Study the drawing (mm; zero at the part's minimum x, y, z) and answer. A direction names the side the tool comes from. Give positions to 0.01 mm unless a question says otherwise; leave off trailing zeros. Write each loop counter-clockwise with the first axis right and the second up, starting at its lowest first coordinate (ties: lowest second). Pieces come first, ordered by that corner, then holes. Notation, with made-up numbers: M 1,10 L 40,10 A14 cw 40,28 Z; hole C -0.75,-25 d11. An arc over 180 degrees is marked long. Use a Markdown table: item, result. Add a question column.
Item 1: Given P1, Ø8, axis at x = 58, z = 9, coming from the -Y side; P2, Ø4, axis at y = 15, z = 13, coming from the -X side, each flat-ended and moving along its own axis, determine where each tip first touches the part or whether it passes through.
Item 2: Consider probe 1 along Z at (x, y) = (50.5, 27); probe 2 along Y at (x, z) = (58.5, 17.75). Determine where each line is inside the solid, lowest interval first. Write a range as [from, to].
Item 3: For the marked faces 1 and 2, determine the directions among +Z, -Z, +X, -X, +Y, -Y from which every point of the face is accessible in a straight line to the end or side of a thin tool.
Item 4: A cutting plane is placed at A-A on y = 44. Determine the outline of the cut face in (x, z).
Item 5: A cutting plane is placed at C-C on x = 31.5. Determine the outline of the cut face in (y, z), then the cut area to 3 significant figures.
Item 6: A cutting plane is placed at B-B on x = 48.5. Determine the outline of the cut face in (y, z) (1 decimal).
Item 7: A cutting plane is placed at D-D on z = 6.5. Determine the outline of the cut face in (x, y), then the cut area to 3 significant figures.
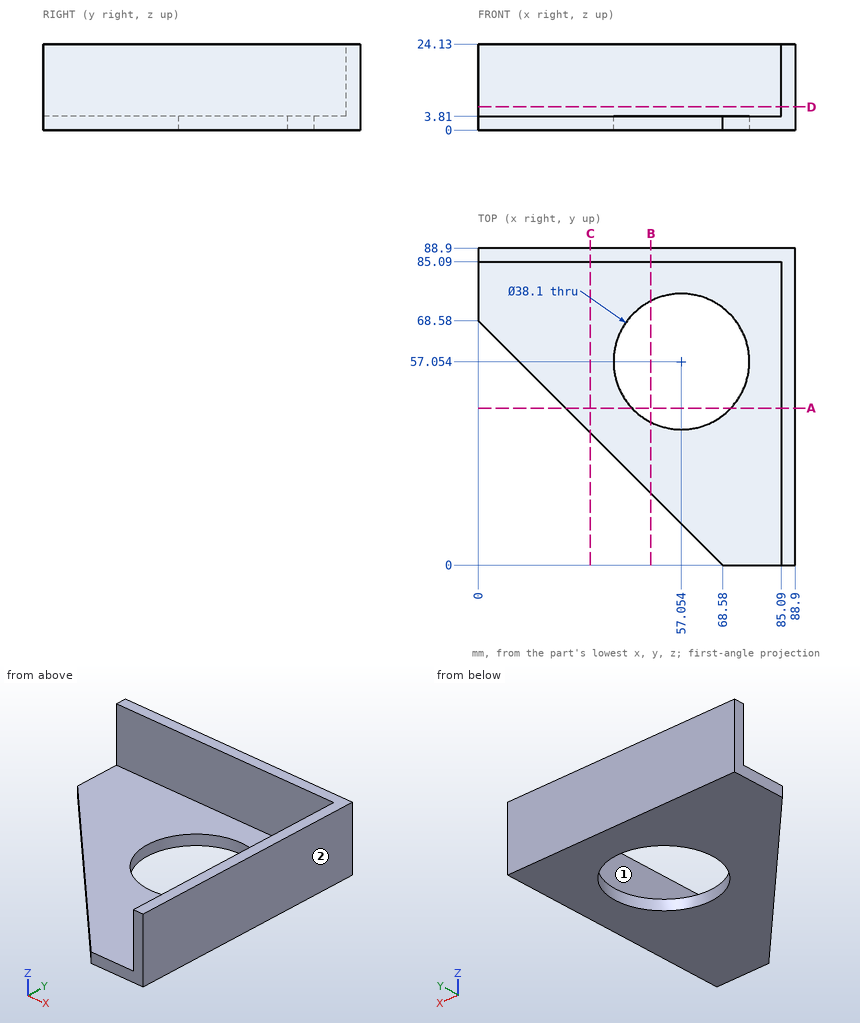
Filled in:
| question | item | result |
|---|---|---|
| 1 | P1 | y = 85.09 |
| 1 | P2 | x = 85.09 |
| 2 | probe 1 | [0, 3.81] |
| 2 | probe 2 | [85.09, 88.9] |
| 3 | face 1 | +Z, -X, -Y |
| 3 | face 2 | +Z, -Z, +X, +Y, -Y |
| 4 | outline | M 24.58,0 L 43.18,0 L 43.18,3.81 L 24.58,3.81 Z; M 70.93,0 L 88.9,0 L 88.9,24.13 L 85.09,24.13 L 85.09,3.81 L 70.93,3.81 Z |
| 5 | outline | M 37.08,0 L 88.9,0 L 88.9,24.13 L 85.09,24.13 L 85.09,3.81 L 37.08,3.81 Z |
| 5 | area | 275 mm² |
| 6 | outline | M 20.1,0 L 40,0 L 40,3.8 L 20.1,3.8 Z; M 74.1,0 L 88.9,0 L 88.9,24.1 L 85.1,24.1 L 85.1,3.8 L 74.1,3.8 Z |
| 7 | outline | M 0,85.09 L 85.09,85.09 L 85.09,0 L 88.9,0 L 88.9,88.9 L 0,88.9 Z |
| 7 | area | 663 mm² |
